For this review, take the finished solid that the model builds, in its own axes (mm). A direction names the side the tool comes from. Give positions to 0.01 mm unless a question says otherwise; leave off trailing zeros. Loops run counter-clockwise (first coordinate to the right, second up) from the corner with the lowest first, then second, coordinate; pieces in that order, holes last. Notation, with made-up numbers: (77, 27.5) - (121, 27.5) arc R21 ccw to (121, 41.5) - close; hole circle Ø7 at (53, -23). An arc over 180 degrees is marked (long way). Answer in a Markdown table with one row per item.
Autodesk Inventor part; units mm, degrees
ref_plane "YZ Plane" through (0, 0, 0) normal (1, 0, 0) x (0, 1, 0)
ref_plane "XZ Plane" through (0, 0, 0) normal (0, 1, 0) x (-1, 0, 0)
ref_plane "XY Plane" through (0, 0, 0) normal (0, 0, 1) x (1, 0, 0)
sketch "スケッチ1" plane through (0, 0, 0) normal (0, 1, 0) x (-1, 0, 0)
  line L0 (3, 0) -> (6, 0)
  line L1 (6, 0) -> (6, 1.5)
  line L2 (6, 1.5) -> (5, 1.5)
  line L3 (5, 1.5) -> (5, 5)
  line L4 (4.5, 6) -> (3, 6)
  line L5 (3, 6) -> (3, 0)
  line L6 (5, 5) -> (4.5, 6)
  line L7 (0, -1.2) -> (0, 7.2)
  point P0 (0, 0)
  point P1 (3, 6)
  dimension "d5" = 1.5
  dimension "d9" = 1
  dimension "d10" = 0.5
  dimension "d17" = 10
  dimension "d18" = 12
  dimension "d19" = 6
  dimension "d20" = 6
revolve "回転1" add sketch "スケッチ1" angle 360 about axis through (0, 0, -10) along (0, 0, 1)
sketch "スケッチ2" plane through (0, 0, 6) normal (0, 0, 1) x (1, 0, 0)
  line L0 (4.4, -2.3749) -> (-4.4, -2.3749)
  line L1 (-4.4, -2.3749) -> (-4.4, 2.3749)
  line L2 (-4.4, 2.3749) -> (4.4, 2.3749)
  line L3 (4.4, 2.3749) -> (4.4, -2.3749)
  line L4 (4.4, -2.3749) -> (-4.4, 2.3749) construction
  line L5 (-4.4, -2.3749) -> (4.4, 2.3749) construction
  circle A0 centre (0, 0) radius 5
  point P0 (0, 0)
  dimension "d12" = 10
  dimension "d11" = 8.8
extrude "押し出し1" cut sketch "スケッチ2" against normal up to surface (4.5 mm away) contours L3 A0 | A0 L1
sketch "스케치3" plane through (0, 0, 6) normal (0, 0, 1) x (1, 0, 0)
  circle A0 centre (0, 0) radius 3
  line L0 (4.4, -0.9434) -> (4.4, 0.9434)
  arc A1 (4.4, 0.9434) -> (-4.4, 0.9434) centre (0, 0) ccw
  line L1 (-4.4, 0.9434) -> (-4.4, -0.9434)
  arc A2 (-4.4, -0.9434) -> (4.4, -0.9434) centre (0, 0) ccw
  circle A3 centre (0, 0) radius 3.025
  dimension "d21" = 6.05
extrude "돌출2" cut sketch "스케치3" against normal up to surface (6 mm away) contours A0 | A3
properties part number "LED-0606" material "アセタール樹脂、黒"
1. For faces 4 (the face through (0, 5, 3)), 5 (the face through (-4.4, 0, 4)), 6 (the face through (4.4, 0, 4)), 7 (the face through (0, -5, 3)), list the 3-axis set-ups (+Z, -Z, +X, -X, +Y, -Y) from which the entire face can be reached by the end or side of a thin tool; tool diameter is ignored.
Values:
| item | result |
|---|---|
| face 4 | +Z, +Y |
| face 5 | +Z, -X, +Y, -Y |
| face 6 | +Z, +X, +Y, -Y |
| face 7 | +Z, -Y |
2. We need section B-B, the plane y = 0. Give the boundary of the cut face in (x, z) (3 decimals), and give its area (3 significant figures).
Values:
| item | result |
|---|---|
| outline | (-6, 0) - (-3.025, 0) - (-3.025, 6) - (-4.4, 6) - (-4.4, 1.5) - (-6, 1.5) - close; (3.025, 0) - (6, 0) - (6, 1.5) - (4.4, 1.5) - (4.4, 6) - (3.025, 6) - close |
| area | 21.3 mm^2 |
3. Clearance check with flat-ended pins moving along their axes: pin 1 (3.5 mm diameter, centred on y = -0.5, z = 3.5, fed in from +X); pin 2 (1.5 mm diameter, centred on y = -4.5, z = 5, fed in from +X); pin 3 (3 mm diameter, centred on x = 4, z = 4, fed in from -Y). State where each tip first meets the part, or that it passes through.
Values:
| item | result |
|---|---|
| pin 1 | stops at x = 4.4 |
| pin 2 | stops at x = 3.31 |
| pin 3 | stops at y = -4.33 |
4. We need section D-D, the plane x = -5. Give the boundary of the cut face in (y, z).
Values:
| item | result |
|---|---|
| outline | (-3.32, 0) - (3.32, 0) - (3.32, 1.5) - (-3.32, 1.5) - close |
5. Mouldability with a two-part tool opening along Y and no side actions: class faces 1 (the face through (2.794, -1.159, 3.042)), 2 (the face through (-0.1, 4.6, 5.8)), 3 (the face through (3, -1.1, 6)) as released by +Y, released by -Y, zero draft, split by the parting line, or undercut.
Values:
| item | result |
|---|---|
| face 1 | undercut |
| face 2 | released by +Y |
| face 3 | zero draft |
6. We need section C-C, the plane z = 5.25. Give the boundary of the cut face in (x, y) (3 decimals), and give its area (3 significant figures).
Values:
| item | result |
|---|---|
| outline | (-4.4, -2.099) arc R4.875 ccw to (4.4, -2.099) - (4.4, 2.099) arc R4.875 ccw to (-4.4, 2.099) - close; hole circle Ø6.05 at (0, 0) |
| area | 43.2 mm^2 |
7. We need section A-A, the plane x = 0. Give the boundary of the cut face in (y, z) (3 decimals).
Values:
| item | result |
|---|---|
| outline | (-6, 0) - (-3.025, 0) - (-3.025, 6) - (-4.5, 6) - (-5, 5) - (-5, 1.5) - (-6, 1.5) - close; (3.025, 0) - (6, 0) - (6, 1.5) - (5, 1.5) - (5, 5) - (4.5, 6) - (3.025, 6) - close |
8. Wall thickness on line 1 (Y direction, x = 0, z = 1.4) (3 decimals); line 2 (Z direction, x = 2.75, y = 5); line 3 (X direction, y = 2.75, z = 3.75): over which ranges is each line inside the solid? List them lowest first. Write a range as [from, to].
Values:
| item | result |
|---|---|
| line 1 | y = [-6, -3.025], [3.025, 6] |
| line 2 | z = [0, 1.5] |
| line 3 | x = [-4.18, -1.26], [1.26, 4.18] |
